Check sheet for the modelled part. Datum: model origin and axes. Units: mm. A direction names the side the tool comes from. Coordinates: 2 decimals unless noted, no trailing zeros. Order: outer loops, then holes, each group sorted by start corner. A loop starts at its lowest first (then second) coordinate and runs counter-clockwise, first axis right, second up.
1. Cross-section at B-B (z = 7.5). Enter the section's corners in (x, y).
2. Cross-section at A-A (y = 26). Enter the section's corners in (x, z).
3. Cross-section at D-D (z = 0). Count the separate pieces of the cut face and the enclosed holes in it, then the cut area to 3 significant figures.
4. Set-up check for faces 1 (the flat face through (14, 22, 1)), 2 (the flat face through (0.4, 17.8, -7)), 3 (the flat face through (-27, 4, -2)), 4 (the flat face through (-4, 27, 5)), 5 (the flat face through (-6.5, 6, 1)): record each of +Z, -Z, +X, -X, +Y, -Y from which the full face is reachable in a straight line by a thin tool's end or side.
5. Cross-section at C-C (x = -8). Enter the section's corners in (y, z), then the cut area to 4 significant figures.
6. Thickness scan on line 1 (X direction, y = 3.25, z = 0); line 2 (X direction, y = 32, z = 0.75); line 3 (Z direction, x = 20, y = 5). Record the ranges inside material, lowest first.
7. Draft check along X on faces 6 (the flat face through (4, 26, 5)), 7 (the flat face through (15, 0, 1)), 8 (the flat face through (-14, 22, 1)). Enter one of: released by +X, released by -X, zero draft, split by the parting line, or undercut.
8. Gauge pin test, flat ends, axial feed: pin 1 Ø1.5 at (x, z) = (-4, -4) entering from -Y; pin 2 Ø5 at (y, z) = (25, 3.5) entering from +X; pin 3 Ø2 at (y, z) = (25.5, 4.5) entering from -X. Record the tip position at first contact, or that the pin passes through.
```python
from build123d import *

# Parameters (mm, degrees)
CROQUIS2_R                = 3.5
SALIENTE_EXTRUIR1_DEPTH   = 9
SALIENTE_EXTRUIR1_2_DEPTH = 9
SALIENTE_EXTRUIR2_DEPTH   = 16
CROQUIS4_R                = 3.5
CORTAR_EXTRUIR1_DEPTH     = 28


with BuildPart() as part:
    # Croquis2 → Saliente-Extruir1 (new body)
    with BuildSketch(Plane(origin=(0, 0, 0), x_dir=(1, 0, 0), z_dir=(0, 1, 0))):
        Polygon((-27, 7), (-27, -3), (-20, -9), (-6.5, -9), (-6.5, 7), align=None)
        with Locations(Location((-20, 0, 0), (0, 0, 270))):
            Circle(CROQUIS2_R, mode=Mode.SUBTRACT)
    extrude(amount=SALIENTE_EXTRUIR1_DEPTH)



with BuildPart() as body_2:
    # Croquis2 → Saliente-Extruir1 2 (new body)
    with BuildSketch(Plane(origin=(0, 0, 0), x_dir=(1, 0, 0), z_dir=(0, 1, 0))):
        Polygon((6.5, 7), (27, 7), (27, -3), (20, -9), (6.5, -9), align=None)
        with Locations(Location((20, 0, 0), (0, 0, 90))):
            Circle(CROQUIS2_R, mode=Mode.SUBTRACT)
    extrude(amount=SALIENTE_EXTRUIR1_2_DEPTH)


with BuildPart() as part_1:
    add(part.part)

    add(body_2.part)  # Saliente-Extruir2 merges body 2
    # Croquis3 → Saliente-Extruir2 (add)
    with BuildSketch(Plane.XY.offset(9)):
        Polygon((6.5, 9), (6.5, 11), (-6.5, 11), (-6.5, 9), (-14, 9), (-14, 35.124101005), (-4, 35.124101005), (-4, 18), (4, 18), (4, 35.124101005), (14, 35.124101005), (14, 9), align=None)
    extrude(amount=-SALIENTE_EXTRUIR2_DEPTH)

    # Croquis4 → Cortar-Extruir1 (cut)
    with BuildSketch(Plane(origin=(14, 0, 0), x_dir=(0, 0, -1), z_dir=(1, 0, 0))):
        with Locations((-1, 26)):
            Circle(CROQUIS4_R)
    extrude(amount=-CORTAR_EXTRUIR1_DEPTH, mode=Mode.SUBTRACT)


solid = part_1.part
```
Data:
1. outline: (-21.75, 0) - (-6.5, 0) - (-6.5, 11) - (6.5, 11) - (6.5, 0) - (21.75, 0) - (21.75, 9) - (14, 9) - (14, 35.12) - (4, 35.12) - (4, 18) - (-4, 18) - (-4, 35.12) - (-14, 35.12) - (-14, 9) - (-21.75, 9) - close
2. outline: (-14, -7) - (-4, -7) - (-4, -2.5) - (-14, -2.5) - close; (-14, 4.5) - (-4, 4.5) - (-4, 9) - (-14, 9) - close; (4, -7) - (14, -7) - (14, -2.5) - (4, -2.5) - close; (4, 4.5) - (14, 4.5) - (14, 9) - (4, 9) - close
3. separate pieces: 5
3. enclosed holes: 0
3. area: 677 mm2
4. face 1: +Z, -Z, +X, +Y
4. face 2: -Z, +X, -X, +Y, -Y
4. face 3: +Z, -Z, -X, +Y, -Y
4. face 4: +Z, -Z, +Y
4. face 5: +Z, -Z, -Y
5. outline: (0, -7) - (35.12, -7) - (35.12, 9) - (0, 9) - close; hole circle Ø7 at (26, 1)
5. area: 523.5 mm2
6. line 1: x = -27 to -23.5, -16.5 to -6.5, 6.5 to 16.5, 23.5 to 27
6. line 2: x = -14 to -4, 4 to 14
6. line 3: z = -7 to -3.5, 3.5 to 9
7. face 6: undercut
7. face 7: zero draft
7. face 8: released by -X
8. pin 1: stops at y = 11
8. pin 2: stops at x = 14
8. pin 3: stops at x = -14
